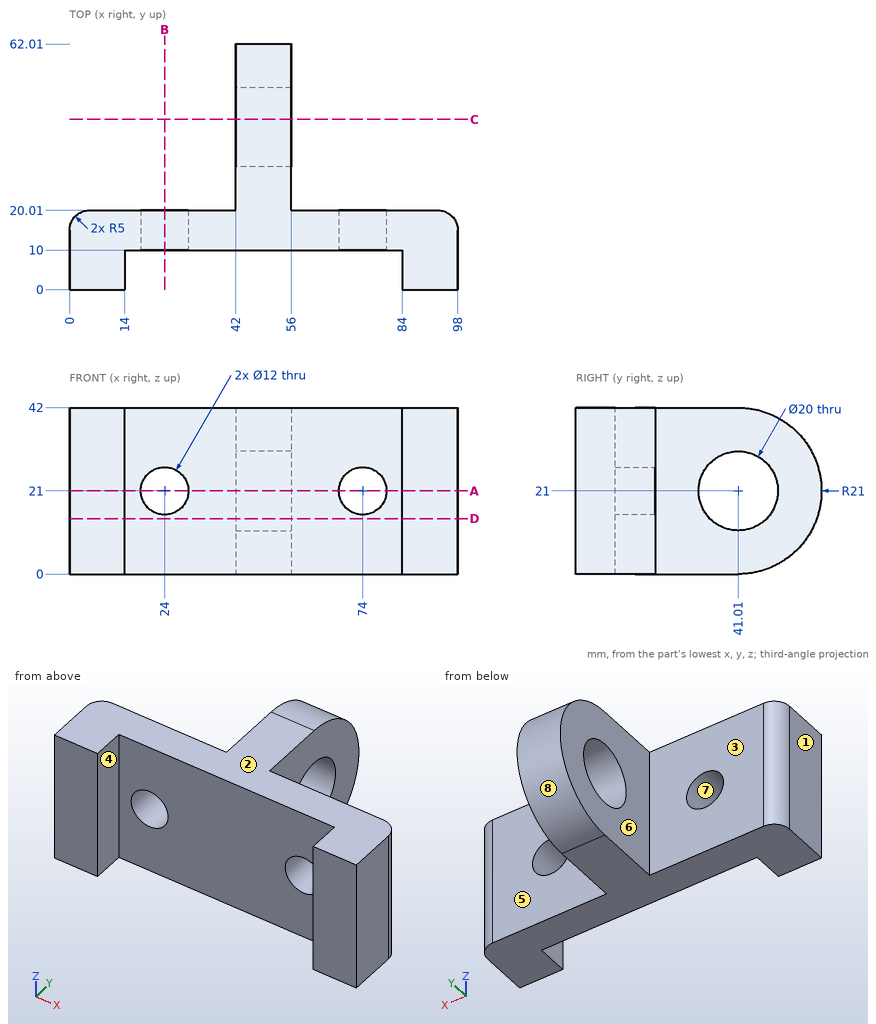
For this review, use the dimensioned drawing (mm, ordinates from the lowest corner) and the shaded views. A direction names the side the tool comes from. Coordinates: 2 decimals unless noted, no trailing zeros. Loops run counter-clockwise (first coordinate to the right, second up) from the corner with the lowest first, then second, coordinate; pieces in that order, holes last. Notation, with made-up numbers: (-20, -29.75) -> (20, -29.75) arc R37 ccw to (20, 9.25) -> close; hole circle Ø6 at (-28, 56). An arc over 180 degrees is marked (long way). Return JSON: item names as keys, results as strings. Group by question number.
(1) Tool access review of the marked faces 1, 2, 3, 4 and 5: name each direction out of +Z, -Z, +X, -X, +Y, -Y from which nothing blocks a thin tool from reaching the whole face with its end or side.
(2) Consider section D-D, the plane z = 14. Give the boundary of the cut face in (x, y).
(3) Consider section B-B, the plane x = 24. Give the boundary of the cut face in (y, z), plus the area to 3 significant figures.
(4) Consider section A-A, the plane z = 21. Give the boundary of the cut face in (x, y).
(5) For pin 1 Ø6 at (y, z) = (52.5, 21) entering from +X; pin 2 Ø23 at (y, z) = (41.01, 21) entering from -X; pin 3 Ø12.5 at (x, z) = (45.5, 31) entering from -Y, all flat-tipped, find the tip position at first contact; note any pin that passes through.
(6) Consider section C-C, the plane y = 43. Give the boundary of the cut face in (x, z), plus the area to 3 significant figures.
(7) To check wall thickness, follow L1, parallel to X at y = 12, z = 21; L2, parallel to X at y = 46.5, z = 10; L3, parallel to Y at x = 51.5, z = 16. State the ranges of each line that lie inside material, in increasing order.
(8) Mouldability with a two-part tool opening along Z and no side actions: class the marked faces 6, 7 and 8 as pulls with the +Z half, pulls with the -Z half, needs draft (parallel to the pull), parting line crosses it, or undercut.
Results below:
{
 "1": {"face 1": "+Z, -Z, -X, +Y, -Y", "face 2": "+Z, +X, -X, +Y, -Y", "face 3": "+Z, -Z, -X, +Y", "face 4": "+Z, -Z, -Y", "face 5": "+Z, -Z, +X, +Y"},
 "2": {"outline": "(0, 0) -> (14, 0) -> (14, 10) -> (84, 10) -> (84, 0) -> (98, 0) -> (98, 15.01) arc R5 ccw to (93, 20.01) -> (56, 20.01) -> (56, 33.87) -> (42, 33.87) -> (42, 20.01) -> (5, 20.01) arc R5 ccw to (0, 15.01) -> close; (42, 48.15) -> (56, 48.15) -> (56, 60.81) -> (42, 60.81) -> close"},
 "3": {"outline": "(10, 0) -> (20.01, 0) -> (20.01, 15) -> (10, 15) -> close; (10, 27) -> (20.01, 27) -> (20.01, 42) -> (10, 42) -> close", "area": "300 mm2"},
 "4": {"outline": "(0, 0) -> (14, 0) -> (14, 10) -> (18, 10) -> (18, 20.01) -> (5, 20.01) arc R5 ccw to (0, 15.01) -> close; (30, 10) -> (68, 10) -> (68, 20.01) -> (56, 20.01) -> (56, 31.01) -> (42, 31.01) -> (42, 20.01) -> (30, 20.01) -> close; (42, 51.01) -> (56, 51.01) -> (56, 62.01) -> (42, 62.01) -> close; (80, 10) -> (84, 10) -> (84, 0) -> (98, 0) -> (98, 15.01) arc R5 ccw to (93, 20.01) -> (80, 20.01) -> close"},
 "5": {"pin 1": "stops at x = 56", "pin 2": "stops at x = 42", "pin 3": "stops at y = 10"},
 "6": {"outline": "(42, 0.09) -> (56, 0.09) -> (56, 11.2) -> (42, 11.2) -> close; (42, 30.8) -> (56, 30.8) -> (56, 41.91) -> (42, 41.91) -> close", "area": "311 mm2"},
 "7": {"L1": "x = 0 to 18, 30 to 68, 80 to 98", "L2": "x = 42 to 56", "L3": "y = 10 to 32.35, 49.67 to 61.41"},
 "8": {"face 6": "needs draft", "face 7": "undercut", "face 8": "parting line crosses it"}
}
